Here's how the part is built. I have some questions about the finished solid (model axes, mm). A direction names the side the tool comes from. Coordinates: 2 decimals unless noted, no trailing zeros. Loops run counter-clockwise (first coordinate to the right, second up) from the corner with the lowest first, then second, coordinate; pieces in that order, holes last. Notation, with made-up numbers: (-8, -23) - (33, -23) arc R28 cw to (33, 11) - close; hole circle Ø7 at (75, 67). An arc over 180 degrees is marked (long way). Use a Markdown table: item, result.
```python
from build123d import *

# Parameters (mm, degrees)
ESBO_O1_W                = 43.8
ESBO_O1_H                = 43.8
ESBO_O1_R                = 1.5
RESSALTO_EXTRUS_O1_DEPTH = 2
ESBO_O2_W                = 23
ESBO_O2_H                = 15.6
RESSALTO_EXTRUS_O2_DEPTH = 26
ESBO_O3_W                = 6.9
ESBO_O3_H                = 10
ESBO_O3_W_2              = 30
ESBO_O3_H_2              = 11.9
RESSALTO_EXTRUS_O3_DEPTH = 12


with BuildPart() as part:
    # Esboço1 → Ressalto-extrusão1 (new body)
    with BuildSketch(Plane(origin=(0, 0, 0), x_dir=(1, 0, 0), z_dir=(0, 1, 0))):
        Rectangle(ESBO_O1_W, ESBO_O1_H)
        with Locations(Location((18.5, 18.5, 0), (0, 0, 270))):
            Circle(ESBO_O1_R, mode=Mode.SUBTRACT)
        with Locations(Location((-18.5, 18.5, 0), (0, 0, 270))):
            Circle(ESBO_O1_R, mode=Mode.SUBTRACT)
        with Locations(Location((18.5, -18.5, 0), (0, 0, 270))):
            Circle(ESBO_O1_R, mode=Mode.SUBTRACT)
        with Locations(Location((-18.5, -18.5, 0), (0, 0, 270))):
            Circle(ESBO_O1_R, mode=Mode.SUBTRACT)
    extrude(amount=RESSALTO_EXTRUS_O1_DEPTH)

    # Esboço2 → Ressalto-extrusão2 (add)
    with BuildSketch(Plane(origin=(0, 2, 0), x_dir=(1, 0, 0), z_dir=(0, 1, 0))):
        with Locations((0, -14.1)):
            Rectangle(ESBO_O2_W, ESBO_O2_H)
    extrude(amount=RESSALTO_EXTRUS_O2_DEPTH)

    # Esboço3 → Ressalto-extrusão3 (add)
    with BuildSketch(Plane(origin=(0, 2, 0), x_dir=(1, 0, 0), z_dir=(0, 1, 0))):
        with Locations((-18.45, 5)):
            Rectangle(ESBO_O3_W, ESBO_O3_H)
        with Locations((18.45, 5)):
            Rectangle(ESBO_O3_W, ESBO_O3_H)
        with Locations((0, 15.95)):
            Rectangle(ESBO_O3_W_2, ESBO_O3_H_2)
        with Locations((0, 5)):
            Rectangle(ESBO_O3_W_2, ESBO_O3_H)
    extrude(amount=RESSALTO_EXTRUS_O3_DEPTH)


solid = part.part
```
Q1. Please list where these lines run through material, in increasing order: L1, parallel to X at y = 0.45, z = 18.5; L2, parallel to Z at x = 1, y = 4.75; L3, parallel to Y at x = 8, z = -14. Write a range as from..to.
Check values:
| item | result |
|---|---|
| L1 | -21.9..-20, -17..17, 20..21.9 |
| L2 | -21.9..0, 6.3..21.9 |
| L3 | 0..14 |
Q2. Which directions (+Z, -Z, +X, -X, +Y, -Y) give clear straight access to the entire face, cutting with the end or side of a thin tool? Please do faces 4 (the face through (-15, 8, -16)), 5 (the face through (0, 8, 0)), 6 (the face through (18, 2, -16)).
Check values:
| item | result |
|---|---|
| face 4 | -Z, -X, +Y |
| face 5 | +X, -X, +Y |
| face 6 | -Z, +X, +Y |
Q3. I want a section at B-B, the plane x = 18.5. Write out the boundary of the cut face in (y, z), then the cut area to 3 significant figures.
Check values:
| item | result |
|---|---|
| outline | (0, -21.9) - (2, -21.9) - (2, -20) - (0, -20) - close; (0, -17) - (2, -17) - (2, -10) - (14, -10) - (14, 0) - (2, 0) - (2, 17) - (0, 17) - close; (0, 20) - (2, 20) - (2, 21.9) - (0, 21.9) - close |
| area | 196 mm^2 |
Q4. I want a section at A-A, the plane y = 7.5. Write out the boundary of the cut face in (x, z).
Check values:
| item | result |
|---|---|
| outline | (-21.9, -10) - (-15, -10) - (-15, -21.9) - (15, -21.9) - (15, -10) - (21.9, -10) - (21.9, 0) - (-21.9, 0) - close; (-11.5, 6.3) - (11.5, 6.3) - (11.5, 21.9) - (-11.5, 21.9) - close |
Q5. If we mould it in two halves opening along Z, with no side actions, what happens to faces 1 (the face through (0, 7, -21.9)), 2 (the face through (19.51, 0.99, 17.39)), 3 (the face through (0, 14, -11))? For each: pulls with the +Z half, pulls with the -Z half, needs draft (parallel to the pull), parting line crosses it, or undercut.
Check values:
| item | result |
|---|---|
| face 1 | pulls with the -Z half |
| face 2 | undercut |
| face 3 | needs draft |
Q6. I want a section at C-C, the plane z = 18.5. Write out the boundary of the cut face in (x, y).
Check values:
| item | result |
|---|---|
| outline | (-21.9, 0) - (-20, 0) - (-20, 2) - (-21.9, 2) - close; (-17, 0) - (17, 0) - (17, 2) - (11.5, 2) - (11.5, 28) - (-11.5, 28) - (-11.5, 2) - (-17, 2) - close; (20, 0) - (21.9, 0) - (21.9, 2) - (20, 2) - close |
Q7. Will these pins go through, and if not, where does the flat tip stop? P1, Ø5.5, axis at x = 20, z = -15, coming from the +Y side; P2, Ø8, axis at y = 19.5, z = 13.5, coming from the +X side; P3, Ø2, axis at x = -17, y = 9.5, coming from the -Z side; P4, Ø5, axis at y = 25, z = 3.5, coming from the +X side.
Check values:
| item | result |
|---|---|
| P1 | y = 2 |
| P2 | x = 11.5 |
| P3 | z = -10 |
| P4 | through |
Q8. I want a section at D-D, the plane z = -11.5. Write out the boundary of the cut face in (x, y), then the cut area to 3 significant figures.
Check values:
| item | result |
|---|---|
| outline | (-21.9, 0) - (21.9, 0) - (21.9, 2) - (15, 2) - (15, 14) - (-15, 14) - (-15, 2) - (-21.9, 2) - close |
| area | 448 mm^2 |
